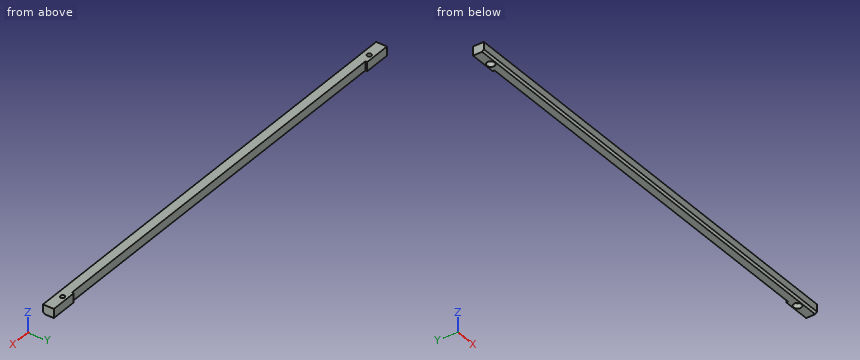
```python
from build123d import *

# Parameters (mm, degrees)
EXTRUDE_1_DEPTH             = 5
CHAMFER_1_SIZE              = 1
HOLE_WIZARD_M21_D           = 2.4
HOLE_WIZARD_M21_CBORE_D     = 4.4
HOLE_WIZARD_M21_CBORE_DEPTH = 2.9


with BuildPart() as part:
    # Эскиз1 → Бобышка-Вытянуть1 (new body)
    with BuildSketch(Plane.XY):
        Polygon((-126, 0), (126, 0), (126, 6), (111, 6), (111, 5), (-111, 5), (-111, 6), (-126, 6), align=None)
    extrude(amount=EXTRUDE_1_DEPTH)

    # Фаска1
    chamfer_1_edges = [part.edges().sort_by_distance(p)[0] for p in [
        (0, 0, 0),
    ]]
    chamfer(chamfer_1_edges, length=CHAMFER_1_SIZE)

    # Цековка для  винта с внутренним шестигранником M21 (through all)
    with Locations(Plane(origin=(0, 0, 0), x_dir=(-1, 0, 0), z_dir=(0, 0, -1))):
        with Locations((-116, 3.5), (116, 3.5)):
            CounterBoreHole(HOLE_WIZARD_M21_D / 2, HOLE_WIZARD_M21_CBORE_D / 2, HOLE_WIZARD_M21_CBORE_DEPTH)


solid = part.part
```
Geometry: final body of the model. Coordinates: model frame, mm. Round coordinates to 2 decimals unless told otherwise and drop trailing zeros. Write each loop counter-clockwise with the first axis right and the second up, starting at its lowest first coordinate (ties: lowest second). Pieces come first, ordered by that corner, then holes.
Item 1: Material intervals for L1, parallel to Y at x = -116, z = 1.15; L2, parallel to X at y = 1.5, z = 1.85; L3, parallel to X at y = 1.75, z = 2.3, sorted ascending.
Item 2: Pin query (flat end, axial travel): P1, Ø3, axis at x = 116, y = 3.5, coming from the +Z side; P2, Ø2, axis at x = -116.5, y = 4.5, coming from the -Z side; P3, Ø1.5, axis at x = 24, z = 2, coming from the +Y side. Return the tip coordinate at first contact, or that it passes through.
Item 3: Section query C-C (x = 5.5). Return loops of the section in (y, z), plus the area to 3 significant figures.
Item 4: Section query A-A (y = 3.5). Return loops of the section in (x, z).
Item 5: Section query B-B (z = 2.15). Return loops of the section in (x, y), plus the area to 3 significant figures.
Completed:
1. L1: y = 0 to 1.3, 5.7 to 6
1. L2: x = -126 to -116.92, -115.08 to 115.08, 116.92 to 126
1. L3: x = -126 to -117.33, -114.67 to 114.67, 117.33 to 126
2. P1: stops at z = 5
2. P2: stops at z = 2.9
2. P3: stops at y = 5
3. outline: (0, 1) - (1, 0) - (5, 0) - (5, 5) - (0, 5) - close
3. area: 24.5 mm2
4. outline: (-126, 0) - (-118.2, 0) - (-118.2, 2.9) - (-117.2, 2.9) - (-117.2, 5) - (-126, 5) - close; (-114.8, 2.9) - (-113.8, 2.9) - (-113.8, 0) - (113.8, 0) - (113.8, 2.9) - (114.8, 2.9) - (114.8, 5) - (-114.8, 5) - close; (117.2, 2.9) - (118.2, 2.9) - (118.2, 0) - (126, 0) - (126, 5) - (117.2, 5) - close
5. outline: (-126, 0) - (126, 0) - (126, 6) - (111, 6) - (111, 5) - (-111, 5) - (-111, 6) - (-126, 6) - close; hole circle Ø4.4 at (-116, 3.5); hole circle Ø4.4 at (116, 3.5)
5. area: 1,260 mm2
